Here's how the part is built. I have some questions about the finished solid (model axes, mm). Round coordinates to 2 decimals unless told otherwise and drop trailing zeros. Loops run counter-clockwise (first coordinate to the right, second up) from the corner with the lowest first, then second, coordinate; pieces in that order, holes last. Notation, with made-up numbers: M 10.5,54.5 L 20.5,54.5 A22 ccw 20.5,64.5 Z; hole C -17,68 d10. An arc over 180 degrees is marked long. Use a Markdown table: item, result.
from build123d import *

# Parameters (mm, degrees)
F0_W     = 90
F0_H     = 57
F0_R     = 1.75
F1_DEPTH = 25


with BuildPart() as f1:
    # F0 (on Top) → F1 (new body)
    with BuildSketch(Plane.XY):
        with Locations((-4, -0.6)):
            Rectangle(F0_W, F0_H)
        with Locations((-9.6017556655, -22.3952072493)):
            Circle(F0_R, mode=Mode.SUBTRACT)
        with BuildLine():
            ThreePointArc((-15.5648804785, -9.1569438638), (-15.5648689141, -9.1606169763), (-15.5648650592, -9.164290105))
            ThreePointArc((-15.5648650592, -9.164290105), (-19.0648612044, -9.1679632337), (-15.5648804785, -9.1569438638))
        make_face(mode=Mode.SUBTRACT)
        with Locations((5.7131093938, -22.3309171443)):
            Circle(F0_R, mode=Mode.SUBTRACT)
        with Locations((13.3148650592, -9.035709895)):
            Circle(F0_R, mode=Mode.SUBTRACT)
        with BuildLine():
            ThreePointArc((4.5, -2.1), (2.5543198547, -6.7376902291), (-2.117898665, -8.5989306739))
            ThreePointArc((-2.117898665, -8.5989306739), (-6.5543198547, 2.5376902291), (4.5, -2.1))
        make_face(mode=Mode.SUBTRACT)
        with Locations((-9.7131093938, 4.1309171443)):
            Circle(F0_R, mode=Mode.SUBTRACT)
        with Locations((5.6017556655, 4.1952072493)):
            Circle(F0_R, mode=Mode.SUBTRACT)
    extrude(amount=F1_DEPTH)


solid = f1.part
1. I need wall thicknesses on probe 1 along X at (y, z) = (-9, 7.25); probe 2 along X at (y, z) = (5.5, 18.5); probe 3 along Y at (x, z) = (13.5, 19.25). Which ranges of each line are inside material? Lowest first, please. Write a range as from..to.
Answer sheet:
| item | result |
|---|---|
| probe 1 | -49..-19.06, -15.57..11.57, 15.06..41 |
| probe 2 | -49..-10.8, -8.62..4.44, 6.77..41 |
| probe 3 | -29.1..-10.78, -7.3..27.9 |
2. Imagine slicing it at A-A, the plane z = 3.25. State how many separate pieces and enclosed holes the cut face has, then the cut area to 3 significant figures.
Answer sheet:
| item | result |
|---|---|
| separate pieces | 1 |
| enclosed holes | 7 |
| area | 4,940 mm2 |
3. Imagine slicing it at C-C, the plane x = -3. Write out the boundary of the cut face in (y, z).
Answer sheet:
| item | result |
|---|---|
| outline | M -29.1,0 L -8.52,0 L -8.52,25 L -29.1,25 Z; M 4.32,0 L 27.9,0 L 27.9,25 L 4.32,25 Z |
4. We'd pull the mould along Y, two halves only. Please class faces 1 (the face through (-5, 27.9, 12)), 2 (the face through (-19.063, -9.245, 12.325)), 3 (the face through (-49, -1, 12)), 4 (the face through (-5, -29.1, 12)): +Y half, -Y half, draft (parallel to the pull), parting line (faces both ways), or undercut.
Answer sheet:
| item | result |
|---|---|
| face 1 | +Y half |
| face 2 | undercut |
| face 3 | draft |
| face 4 | -Y half |
5. Imagine slicing it at B-B, the plane y = -3.5. Write out the boundary of the cut face in (x, z), then the cut area to 3 significant figures.
Answer sheet:
| item | result |
|---|---|
| outline | M -49,0 L -8.35,0 L -8.35,25 L -49,25 Z; M 4.35,0 L 41,0 L 41,25 L 4.35,25 Z |
| area | 1,930 mm2 |
6. For pin 1 Ø17 at (x, y) = (-2, -2.1) entering from +Z, with a flat end and sliding along its axis, tell me the tip position at first contact or that it passes through.
Answer sheet:
| item | result |
|---|---|
| pin 1 | z = 25 |
